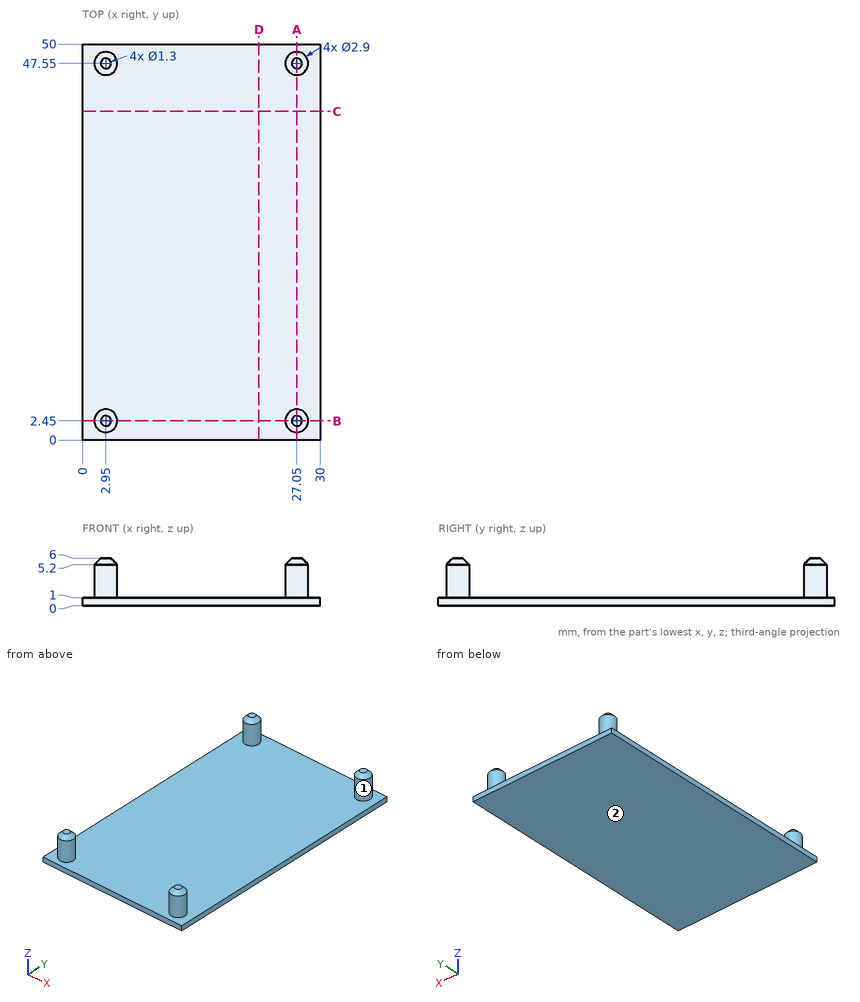
Job drawing, mm, ordinate dimensions from the low corner. One solid piece. Round coordinates to 2 decimals unless told otherwise and drop trailing zeros. Write each loop counter-clockwise with the first axis right and the second up, starting at its lowest first coordinate (ties: lowest second). Pieces come first, ordered by that corner, then holes. Notation, with made-up numbers: (-7, -25) -> (34, -25) arc R21 cw to (34, -2) -> close; hole circle Ø11 at (37.25, 69.5). An arc over 180 degrees is marked (long way). Answer as CSV lines item,"result".
1. Slice it at A-A, the plane x = 27.05. List the corners of the cut face in (y, z), plus the area to 3 significant figures.
Resolved:
outline,"(0, 0) -> (50, 0) -> (50, 1) -> (49, 1) -> (49, 5.2) -> (48.2, 6) -> (46.9, 6) -> (46.1, 5.2) -> (46.1, 1) -> (3.9, 1) -> (3.9, 5.2) -> (3.1, 6) -> (1.8, 6) -> (1, 5.2) -> (1, 1) -> (0, 1) -> close"
area,"77.7 mm²"
2. Pin check, flat tip, straight feed: pin 1 Ø5 at (x, y) = (11, 31.5) entering from +Z. Stop position of the tip, or through.
Resolved:
pin 1,"z = 1"
3. Slice it at C-C, the plane y = 41.5. List the corners of the cut face in (x, z).
Resolved:
outline,"(0, 0) -> (30, 0) -> (30, 1) -> (0, 1) -> close"
4. Slice it at D-D, the plane x = 22.25. List the corners of the cut face in (y, z), plus the area to 3 significant figures.
Resolved:
outline,"(0, 0) -> (50, 0) -> (50, 1) -> (0, 1) -> close"
area,"50.0 mm²"
5. Mould opens along Y. For the marked faces 1 and 2 say: +Y half, -Y half, draft (parallel to the pull), parting line (faces both ways), or undercut.
Resolved:
face 1,"undercut"
face 2,"draft"
6. Drill centre lines: line 1 (Y direction, x = 4.25, z = 3.75); line 2 (Z direction, x = 11.5, y = 44.5); line 3 (Y direction, x = 27.5, z = 2.5). Where is each one in solid material? Low to high.
Resolved:
line 1,"1.81 to 3.09, 46.91 to 48.19"
line 2,"0 to 1"
line 3,"1.07 to 3.83, 46.17 to 48.93"
7. Slice it at B-B, the plane y = 2.45. List the corners of the cut face in (x, z), plus the area to 3 significant figures.
Resolved:
outline,"(0, 0) -> (30, 0) -> (30, 1) -> (28.5, 1) -> (28.5, 5.2) -> (27.7, 6) -> (26.4, 6) -> (25.6, 5.2) -> (25.6, 1) -> (4.4, 1) -> (4.4, 5.2) -> (3.6, 6) -> (2.3, 6) -> (1.5, 5.2) -> (1.5, 1) -> (0, 1) -> close"
area,"57.7 mm²"
